Part print with two shaded views. Sizes in mm from the minimum x, y, z corner. Coordinates: 2 decimals unless noted, no trailing zeros. Loops run counter-clockwise (first coordinate to the right, second up) from the corner with the lowest first, then second, coordinate; pieces in that order, holes last. Notation, with made-up numbers: M 26,-5.5 L 50,-5.5 A30 ccw 50,17.5 Z; hole C -15,63 d3. An arc over 180 degrees is marked long. Use CSV: the item, a comma, the result in double quotes. Start each with the question number.
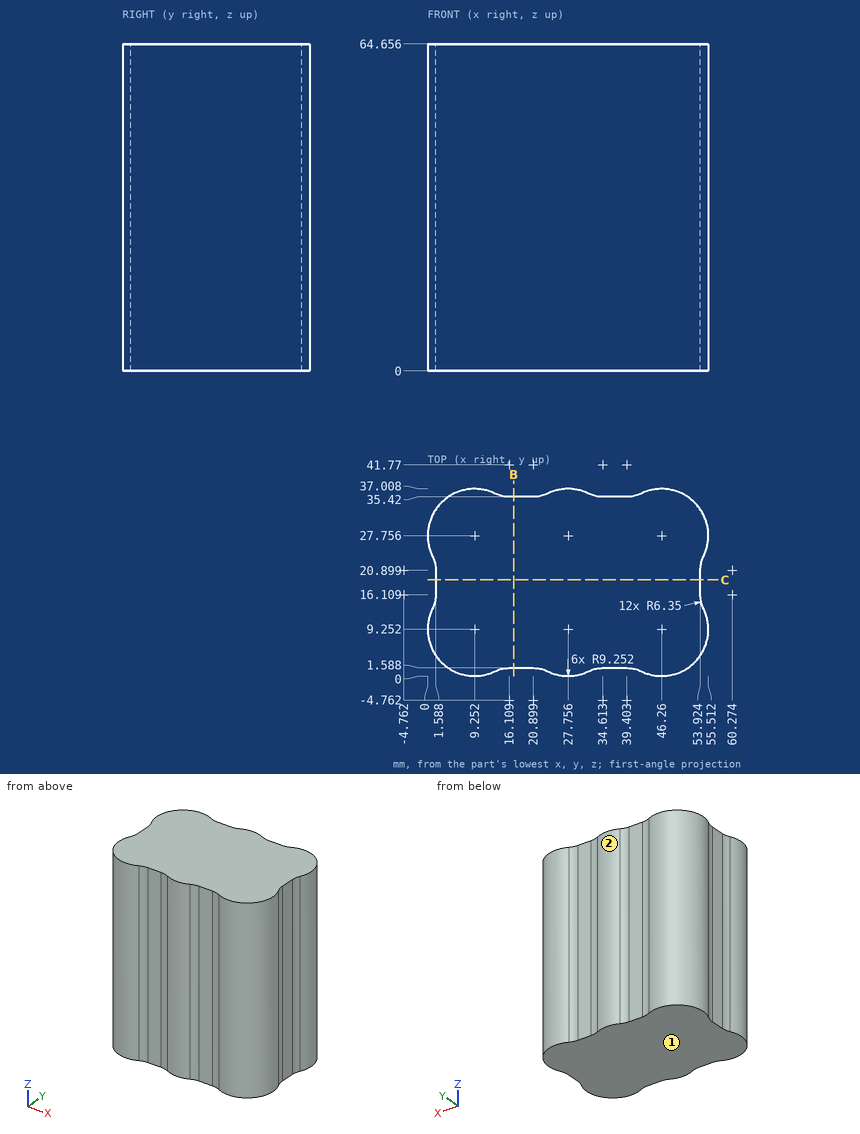
1. Slice it at C-C, the plane y = 19. List the corners of the cut face in (x, z) (1 decimal), and give its area (3 significant figures).
2. Slice it at B-B, the plane x = 17. List the corners of the cut face in (y, z) (1 decimal), and give its area (3 significant figures).
3. Pin check, flat tips, straight feed: pin 1 (1 mm diameter, centred on x = 25, z = 55.5, fed in from +Y); pin 2 (2.5 mm diameter, centred on x = 19, z = 31, fed in from -Y); pin 3 (10 mm diameter, centred on y = 19.5, z = 50.5, fed in from -X). Stop position of each tip, or through.
4. Wall check: probe 1 along Y at (x, z) = (20, 29); probe 2 along X at (y, z) = (13, 41) (1 decimal); probe 3 along X at (y, z) = (19, 28) (1 decimal). Give the ranges that are in metal, low to high.
5. Two-plate mould, pull along X, no slides. Class the marked faces 1 and 2: pulls with the +X half, pulls with the -X half, needs draft (parallel to the pull), parting line crosses it, or undercut.
Found:
1,outline,"M 1.6,0 L 53.9,0 L 53.9,64.7 L 1.6,64.7 Z"
1,area,"3,380 mm^2"
2,outline,"M 1.6,0 L 35.4,0 L 35.4,64.7 L 1.6,64.7 Z"
2,area,"2,190 mm^2"
3,pin 1,"y = 36.73"
3,pin 2,"y = 1.59"
3,pin 3,"x = 0.59"
4,probe 1,"1.59 to 35.42"
4,probe 2,"0.8 to 54.7"
4,probe 3,"1.6 to 53.9"
5,face 1,"needs draft"
5,face 2,"undercut"
